Verification items for the finished model (mm, model axes). Face numbers are marked on the shaded views. A direction names the side the tool comes from. Give positions to 0.01 mm unless a question says otherwise; leave off trailing zeros. Loops run counter-clockwise (first coordinate to the right, second up) from the corner with the lowest first, then second, coordinate; pieces in that order, holes last. Notation, with made-up numbers: (-1, 83) - (35, 83) arc R22 cw to (35, 105) - close; hole circle Ø11 at (-20.75, 20.5). An arc over 180 degrees is marked (long way). One line per question, with ' | ' between items. Start each with the question number.
1. Depth check by flat-ended pin: pin 1 Ø4.5 at (x, y) = (-12, 2.5) entering from +Z; pin 2 Ø4.5 at (y, z) = (0, 9.5) entering from +X; pin 3 Ø1.5 at (y, z) = (-6.5, 2.5) entering from +X; pin 4 Ø2.5 at (x, y) = (11.7, -3.3) entering from +Z. Enter the tip coordinate at first touch or a pass-through.
2. Thickness scan on line 1 along X through (y, z) = (0.5, 9); line 2 along Y through (x, z) = (11.7, 0.85); line 3 along Y through (x, z) = (-11.7, 0.8). Record the ranges inside material, lowest first. Write a range as from..to.
3. Section check C-C, the plane y = -2.5. Enter the section's corners in (x, z).
4. Section check A-A, the plane z = 2.75. Enter the section's corners in (x, y), then the cut area to 3 significant figures.
5. Section check D-D, the plane x = 11.5. Enter the section's corners in (y, z), then the cut area to 3 significant figures.
6. Tool access check on the marked faces 4, 5, 6 and 7. Record the directions out of +Z, -Z, +X, -X, +Y, -Y that give a thin tool (end or side, any length) a straight path to the whole face; none if there is none.
7. Mould release check, pull along X, two halves, no side actions. Record for the marked faces 1, 2 and 3: +X half, -X half, draft (parallel to the pull), parting line (faces both ways), or undercut.
8. Section check B-B, the plane x = 6.5. Enter the section's corners in (y, z).
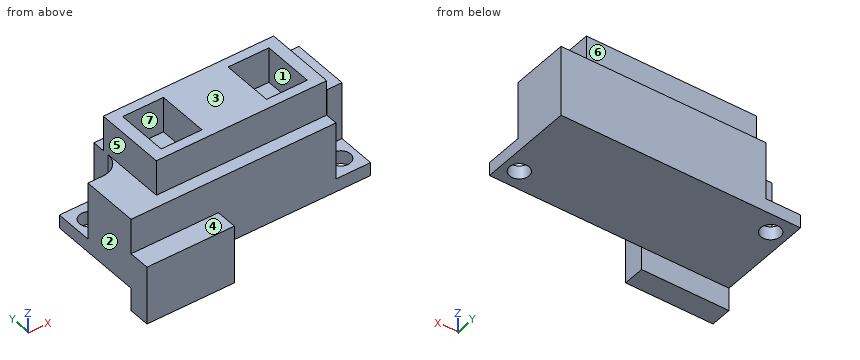
from build123d import *

# Parameters (mm, degrees)
SKETCH1_W                = 27
SKETCH1_H                = 10.8
BOSS_EXTRUDE1_DEPTH      = 12
SKETCH2_R                = 1.1
CUT_EXTRUDE1_DEPTH       = 19.852320812
CUT_EXTRUDE2_DEPTH       = 10.5
SKETCH4_W                = 27
SKETCH4_H                = 10.8
SKETCH4_W_2              = 19.2
SKETCH4_H_2              = 8
CUT_EXTRUDE3_DEPTH       = 4
SKETCH5_W                = 4.6
SKETCH5_H                = 5.8
CUT_EXTRUDE4_DEPTH       = 4
BOSS_EXTRUDE2_DEPTH      = 2.6
BOSS_EXTRUDE2_DEPTH_BACK = 4
SKETCH7_W                = 9.85
SKETCH7_H                = 2.4


with BuildPart() as part:
    # Sketch1 → Boss-Extrude1 (new body)
    with BuildSketch(Plane.XY):
        Rectangle(SKETCH1_W, SKETCH1_H)
    extrude(amount=BOSS_EXTRUDE1_DEPTH)

    # Sketch2 → Cut-Extrude1 (cut, through all)
    with BuildSketch(Plane.XY.offset(12)):
        with Locations((-11.7, 3.3)):
            Circle(SKETCH2_R)
        with Locations((11.7, -3.3)):
            Circle(SKETCH2_R)
    extrude(amount=-CUT_EXTRUDE1_DEPTH, mode=Mode.SUBTRACT)

    # Sketch3 → Cut-Extrude2 (cut)
    with BuildSketch(Plane.XY.offset(12)):
        with BuildLine():
            Line((9.6, -5.4), (9.6, -3.3))
            ThreePointArc((9.6, -3.3), (10.244365081, -1.744365081), (11.8, -1.1))
            Line((11.8, -1.1), (13.5, -1.1))
            Line((13.5, -1.1), (13.5, -5.4))
            Line((13.5, -5.4), (9.6, -5.4))
        make_face()
        with BuildLine():
            Line((-9.6, 5.4), (-9.6, 3.3))
            ThreePointArc((-9.6, 3.3), (-10.244365081, 1.744365081), (-11.8, 1.1))
            Line((-11.8, 1.1), (-13.5, 1.1))
            Line((-13.5, 1.1), (-13.5, 5.4))
            Line((-13.5, 5.4), (-9.6, 5.4))
        make_face()
    extrude(amount=-CUT_EXTRUDE2_DEPTH, mode=Mode.SUBTRACT)

    # Sketch4 → Cut-Extrude3 (cut)
    with BuildSketch(Plane.XY.offset(12)):
        Rectangle(SKETCH4_W, SKETCH4_H)
        Rectangle(SKETCH4_W_2, SKETCH4_H_2, mode=Mode.SUBTRACT)
    extrude(amount=-CUT_EXTRUDE3_DEPTH, mode=Mode.SUBTRACT)

    # Sketch5 → Cut-Extrude4 (cut)
    with BuildSketch(Plane.XY.offset(12)):
        with Locations((-5.94, 0)):
            Rectangle(SKETCH5_W, SKETCH5_H)
        with Locations((5.94, 0)):
            Rectangle(SKETCH5_W, SKETCH5_H)
    extrude(amount=-CUT_EXTRUDE4_DEPTH, mode=Mode.SUBTRACT)

    # Sketch7 → Boss-Extrude2 (add, two sides: drawn at the far end of the back side and taken through both)
    with BuildSketch(Plane(origin=(0, 0, 0), x_dir=(-1, 0, 0), z_dir=(0, 0, -1)).offset(-BOSS_EXTRUDE2_DEPTH_BACK)):
        with Locations((8.575, -6.6)):
            Rectangle(SKETCH7_W, SKETCH7_H)
    extrude(amount=BOSS_EXTRUDE2_DEPTH + BOSS_EXTRUDE2_DEPTH_BACK)


solid = part.part
Results list:
1) pin 1: z = 8 | pin 2: x = 13.5 | pin 3: x = -3.65 | pin 4: z = 1.5
2) line 1: -9.6..-8.24, -3.64..3.64, 8.24..9.6 | line 2: -5.4..-4.4, -2.2..5.4 | line 3: -7.8..2.2, 4.4..5.4
3) outline: (-13.5, 0) - (10.95, 0) - (10.95, 1.5) - (9.75, 1.5) - (9.75, 8) - (9.6, 8) - (9.6, 12) - (8.24, 12) - (8.24, 8) - (3.64, 8) - (3.64, 12) - (-3.64, 12) - (-3.64, 8) - (-8.24, 8) - (-8.24, 12) - (-9.6, 12) - (-9.6, 8) - (-13.5, 8) - close; (12.45, 0) - (13.5, 0) - (13.5, 1.5) - (12.45, 1.5) - close
4) outline: (-13.5, -7.8) - (-3.65, -7.8) - (-3.65, -5.4) - (9.6, -5.4) - (9.6, -3.3) arc R2.2 cw to (11.8, -1.1) - (13.5, -1.1) - (13.5, 5.4) - (-9.6, 5.4) - (-9.6, 3.3) arc R2.2 cw to (-11.8, 1.1) - (-13.5, 1.1) - close | area: 284 mm²
5) outline: (-5.4, 0) - (-4.38, 0) - (-4.38, 1.5) - (-5.4, 1.5) - close; (-2.22, 0) - (5.4, 0) - (5.4, 8) - (-1.12, 8) - (-1.12, 1.5) - (-2.22, 1.5) - close | area: 55.3 mm²
6) face 4: +Z, +X, -X, -Y | face 5: +Z, -X, +Y | face 6: +Z, +X, -X, +Y | face 7: +Z
7) face 1: undercut | face 2: -X half | face 3: draft
8) outline: (-5.4, 0) - (5.4, 0) - (5.4, 8) - (4, 8) - (4, 12) - (2.9, 12) - (2.9, 8) - (-2.9, 8) - (-2.9, 12) - (-4, 12) - (-4, 8) - (-5.4, 8) - close
